For this review, take the finished solid that the model builds, in its own axes (mm). A direction names the side the tool comes from. Coordinates: 2 decimals unless noted, no trailing zeros. Order: outer loops, then holes, each group sorted by start corner. A loop starts at its lowest first (then second) coordinate and runs counter-clockwise, first axis right, second up. Notation, with made-up numbers: (59.5, 5) -> (83.5, 5) arc R21 ccw to (83.5, 13) -> close; hole circle Ø11 at (36, 48.5). An arc over 180 degrees is marked (long way). Return JSON: item names as keys, results as strings. Group by question number.
Item 1: Machinability: for faces 4 (the flat face through (-40.882, -4, 8)), 5 (the cylindrical face through (-23.322, 31.193, 8.542)), which of the approach directions +Z, -Z, +X, -X, +Y, -Y give a long, thin tool a straight path to every point of the face, cutting with its end or side? Answer none if there is none.
Item 2: For line 1 along X through (y, z) = (-37.75, 8); line 2 along X through (y, z) = (11.5, 7.25); line 3 along Y through (x, z) = (-1, 11.75), list the stretches that pass through material, from the lowest coordinate up.
Item 3: Take a section at C-C (z = 8). Count the separate pieces of the cut face and the enclosed holes in it, then the cut area to 3 significant figures.
Item 4: Insertion check: pin 1 (6 mm diameter, centred on y = 8.73, z = 8, fed in from -X); pin 2 (6 mm diameter, centred on x = -19.5, y = -2, fed in from +Z); pin 3 (3 mm diameter, centred on x = -20.88, z = 8, fed in from -Y). Each pin has a flat end and moves straight along its axis. Give the tip position at first contact, or say it passes through.
Item 5: Draft analysis for pull direction X (two halves, no side actions). For faces 1 (the flat face through (49.118, -4, 8)), 2 (the flat face through (-45.882, -4, 6)), 3 (the flat face through (4, -37, 13)), state which applies: +X half, -X half, draft (parallel to the pull), parting line (faces both ways), or undercut.
Item 6: Take a section at A-A (x = 13). Write out the cut boundary in (y, z).
Item 7: Take a section at B-B (y = -22). Write out the cut boundary in (x, z).
```python
from build123d import *

# Parameters (mm, degrees)
BOSS_EXTRU_1_DEPTH        = 13
COQUE1_T                  = -5
COQUE1_THICKNESS_2_FACE_W = 90
COQUE1_THICKNESS_2_FACE_H = 65
COQUE1_THICKNESS_2_DEPTH  = 2
ENL_V_MAT_EXTRU_1_REACH   = 110.96
ESQUISSE2_R               = 2.5
ENL_V_MAT_EXTRU_2_REACH   = 95.396
ESQUISSE3_R               = 2.5
BOSS_EXTRU_2_DEPTH        = 10


with BuildPart() as part:
    # Esquisse1 → Boss.-Extru.1 (new body)
    with BuildSketch(Plane.XY):
        Polygon((44.118436308, 33.728448276), (54.118436308, 33.728448276), (54.118436308, 23.728448276), (54.118436308, -41.271551724), (-45.881563692, -41.271551724), (-45.881563692, 33.728448276), align=None)
    extrude(amount=BOSS_EXTRU_1_DEPTH)

    # Coque1
    coque1_openings = [part.faces().sort_by_distance(p)[0] for p in [
        (4.118436308, -3.771551724, 13),
    ]]
    offset(amount=COQUE1_T, openings=coque1_openings, kind=Kind.INTERSECTION)

    # Coque1 thickness 2 face (on inner face of the shell) → Coque1 thickness 2 (cut)
    with BuildSketch(Plane(origin=(4.118436308, -3.771551724, 5), x_dir=(-1, 0, 0), z_dir=(0, 0, -1))):
        Rectangle(COQUE1_THICKNESS_2_FACE_W, COQUE1_THICKNESS_2_FACE_H)
    extrude(amount=COQUE1_THICKNESS_2_DEPTH, mode=Mode.SUBTRACT)

    # Enlèv. mat.-Extru.1: up to this face of the body (flat: up to its plane)
    enl_v_mat_extru_1_end = Plane(part.part.faces().sort_by_distance((54.118436308, -3.771551724, 6.5))[0])
    # Esquisse2 → Enlèv. mat.-Extru.1 (cut, up to the picked face)
    with BuildSketch(Plane.ZY.offset(45.881563692), mode=Mode.PRIVATE) as enl_v_mat_extru_1_sk1:
        with Locations(Location((8, -16.271551724, 0), (0, 0, 270))):
            Circle(ESQUISSE2_R)
    enl_v_mat_extru_1_tool1 = split(extrude(enl_v_mat_extru_1_sk1.sketch, amount=-ENL_V_MAT_EXTRU_1_REACH, mode=Mode.PRIVATE), bisect_by=enl_v_mat_extru_1_end, keep=Keep.BOTH, mode=Mode.PRIVATE)
    # Esquisse2 → Enlèv. mat.-Extru.1 (cut, up to the picked face)
    with BuildSketch(Plane.ZY.offset(45.881563692), mode=Mode.PRIVATE) as enl_v_mat_extru_1_sk2:
        with Locations(Location((8, 8.728448276, 0), (0, 0, 270))):
            Circle(ESQUISSE2_R)
    enl_v_mat_extru_1_tool2 = split(extrude(enl_v_mat_extru_1_sk2.sketch, amount=-ENL_V_MAT_EXTRU_1_REACH, mode=Mode.PRIVATE), bisect_by=enl_v_mat_extru_1_end, keep=Keep.BOTH, mode=Mode.PRIVATE)
    add(enl_v_mat_extru_1_tool1.solids().sort_by(Axis((-45.881564, -16.271552, 8), (1, 0, 0)))[0], mode=Mode.SUBTRACT)
    add(enl_v_mat_extru_1_tool2.solids().sort_by(Axis((-45.881564, 8.728448, 8), (1, 0, 0)))[0], mode=Mode.SUBTRACT)

    # Enlèv. mat.-Extru.2: up to this face of the body (flat: up to its plane)
    enl_v_mat_extru_2_end = Plane(part.part.faces().sort_by_distance((4.118436308, 33.728448276, 6.5))[0])
    # Esquisse3 → Enlèv. mat.-Extru.2 (cut, up to the picked face)
    with BuildSketch(Plane.XZ.offset(41.271551724), mode=Mode.PRIVATE) as enl_v_mat_extru_2_sk1:
        with Locations(Location((-20.881563692, 8, 0), (0, 0, 270))):
            Circle(ESQUISSE3_R)
    enl_v_mat_extru_2_tool1 = split(extrude(enl_v_mat_extru_2_sk1.sketch, amount=-ENL_V_MAT_EXTRU_2_REACH, mode=Mode.PRIVATE), bisect_by=enl_v_mat_extru_2_end, keep=Keep.BOTH, mode=Mode.PRIVATE)
    # Esquisse3 → Enlèv. mat.-Extru.2 (cut, up to the picked face)
    with BuildSketch(Plane.XZ.offset(41.271551724), mode=Mode.PRIVATE) as enl_v_mat_extru_2_sk2:
        with Locations(Location((29.118436308, 8, 0), (0, 0, 270))):
            Circle(ESQUISSE3_R)
    enl_v_mat_extru_2_tool2 = split(extrude(enl_v_mat_extru_2_sk2.sketch, amount=-ENL_V_MAT_EXTRU_2_REACH, mode=Mode.PRIVATE), bisect_by=enl_v_mat_extru_2_end, keep=Keep.BOTH, mode=Mode.PRIVATE)
    add(enl_v_mat_extru_2_tool1.solids().sort_by(Axis((-20.881564, -41.271552, 8), (0, 1, 0)))[0], mode=Mode.SUBTRACT)
    add(enl_v_mat_extru_2_tool2.solids().sort_by(Axis((29.118436, -41.271552, 8), (0, 1, 0)))[0], mode=Mode.SUBTRACT)

    # Esquisse4 → Boss.-Extru.2 (add)
    with BuildSketch(Plane.XY.offset(3)):
        Polygon((-30.881563692, 28.728448276), (-40.881563692, 18.728448276), (-40.881563692, 28.728448276), align=None)
        Polygon((49.118436308, 28.728448276), (49.118436308, 18.728448276), (39.118436308, 28.728448276), align=None)
        Polygon((49.118436308, -36.271551724), (49.118436308, -26.271551724), (39.118436308, -36.271551724), align=None)
        Polygon((-30.881563692, -36.271551724), (-40.881563692, -26.271551724), (-40.881563692, -36.271551724), align=None)
    extrude(amount=BOSS_EXTRU_2_DEPTH)


solid = part.part
```
Findings below:
{
 "1": {"face 4": "+Z", "face 5": "+Y, -Y"},
 "2": {"line 1": "x = -45.88 to -23.38, -18.38 to 26.62, 31.62 to 54.12", "line 2": "x = -45.88 to -40.88, 49.12 to 54.12", "line 3": "y = -41.27 to -36.27, 28.73 to 33.73"},
 "3": {"separate pieces": "8", "enclosed holes": "0", "area": "1,650 mm2"},
 "4": {"pin 1": "stops at x = -45.88", "pin 2": "stops at z = 3", "pin 3": "passes through"},
 "5": {"face 1": "undercut", "face 2": "-X half", "face 3": "draft"},
 "6": {"outline": "(-41.27, 0) -> (33.73, 0) -> (33.73, 13) -> (28.73, 13) -> (28.73, 3) -> (-36.27, 3) -> (-36.27, 13) -> (-41.27, 13) -> close"},
 "7": {"outline": "(-45.88, 0) -> (54.12, 0) -> (54.12, 13) -> (49.12, 13) -> (49.12, 3) -> (-40.88, 3) -> (-40.88, 13) -> (-45.88, 13) -> close"}
}
